```python
from build123d import *

# Parameters (mm, degrees)
SKETCH1_R           = 27
BOSS_EXTRUDE1_DEPTH = 5
SKETCH2_R           = 10
BOSS_EXTRUDE2_DEPTH = 2.5
CUT_EXTRUDE1_DEPTH  = 9


with BuildPart() as part:
    # Sketch1 → Boss-Extrude1 (new, symmetric)
    with BuildSketch(Plane.XY):
        Circle(SKETCH1_R)
    extrude(amount=BOSS_EXTRUDE1_DEPTH, both=True)

    # Sketch2 → Boss-Extrude2 (add)
    with BuildSketch(Plane(origin=(0, 0, -5), x_dir=(-1, 0, 0), z_dir=(0, 0, -1))):
        Circle(SKETCH2_R)
    extrude(amount=BOSS_EXTRUDE2_DEPTH)

    # Sketch3 → Cut-Extrude1 (cut)
    with BuildSketch(Plane(origin=(0, 0, -7.5), x_dir=(-1, 0, 0), z_dir=(0, 0, -1))):
        with BuildLine():
            Line((-1.953362486, -1.9), (1.953362486, -1.9))
            ThreePointArc((1.953362486, -1.9), (2.725, 0), (1.953362486, 1.9))
            Line((1.953362486, 1.9), (-1.953362486, 1.9))
            ThreePointArc((-1.953362486, 1.9), (-2.725, 0), (-1.953362486, -1.9))
        make_face()
    extrude(amount=-CUT_EXTRUDE1_DEPTH, mode=Mode.SUBTRACT)


solid = part.part
```
Check sheet for the modelled part. Datum: model origin and axes. Units: mm. A direction names the side the tool comes from. Round coordinates to 2 decimals unless told otherwise and drop trailing zeros. Order: outer loops, then holes, each group sorted by start corner. A loop starts at its lowest first (then second) coordinate and runs counter-clockwise, first axis right, second up. Notation, with made-up numbers: M -26.75,-0.75 L -3.75,-0.75 A20 ccw -3.75,25.25 Z; hole C 85.25,38.25 d6. An arc over 180 degrees is marked long. Answer in a Markdown table with one row per item.
(1) Draft check along Y on faces 3 (the flat face through (12, 0, -5)), 4 (the cylindrical face through (2.725, 0.029, -3.063)), 5 (the cylindrical face through (-5.85, -26.36, 0.07)). Enter one of: +Y half, -Y half, draft (parallel to the pull), parting line (faces both ways), or undercut.
Findings:
| item | result |
|---|---|
| face 3 | draft |
| face 4 | undercut |
| face 5 | parting line |
(2) Material ranges on line 1 along Z through (x, y) = (1.5, 10.5); line 2 along Y through (x, z) = (2, -3.5); line 3 along Y through (x, z) = (-1.5, -6), recorded low to high. Write a range as from..to.
Findings:
| item | result |
|---|---|
| line 1 | z = -5..5 |
| line 2 | y = -26.93..-1.85, 1.85..26.93 |
| line 3 | y = -9.89..-1.9, 1.9..9.89 |
(3) Section check A-A on z = -4.25. Record the boundary of the cut face in (x, y) (3 decimals), plus the area to 3 significant figures.
Findings:
| item | result |
|---|---|
| outline | C 0,0 d54; hole M -1.953,-1.9 L 1.953,-1.9 A2.725 ccw 1.953,1.9 L -1.953,1.9 A2.725 ccw Z |
| area | 2,270 mm^2 |
(4) Set-up check for faces 1 (the flat face through (0.1, -2.1, -7.5)), 2 (the flat face through (0, -1.9, -3)): record each of +Z, -Z, +X, -X, +Y, -Y from which the full face is reachable in a straight line by a thin tool's end or side.
Findings:
| item | result |
|---|---|
| face 1 | -Z, +X, -X, +Y, -Y |
| face 2 | -Z |
(5) Gauge pin test, flat ends, axial feed: pin 1 (4.5 mm diameter, centred on x = 0, z = -3.5, fed in from -Y); pin 2 (5 mm diameter, centred on x = -10, z = 0.5, fed in from -Y); pin 3 (6 mm diameter, centred on x = -13, z = 0, fed in from +Y). Record the tip position at first contact, or that the pin passes through.
Findings:
| item | result |
|---|---|
| pin 1 | stops at y = -27 |
| pin 2 | stops at y = -25.94 |
| pin 3 | stops at y = 25.08 |
(6) Section check B-B on y = 0. Record the boundary of the cut face in (x, z) (3 decimals), plus the area to 3 significant figures.
Findings:
| item | result |
|---|---|
| outline | M -27,-5 L -10,-5 L -10,-7.5 L -2.725,-7.5 L -2.725,1.5 L 2.725,1.5 L 2.725,-7.5 L 10,-7.5 L 10,-5 L 27,-5 L 27,5 L -27,5 Z |
| area | 541 mm^2 |
(7) Section check C-C on x = 0. Record the boundary of the cut face in (y, z).
Findings:
| item | result |
|---|---|
| outline | M -27,-5 L -10,-5 L -10,-7.5 L -1.9,-7.5 L -1.9,1.5 L 1.9,1.5 L 1.9,-7.5 L 10,-7.5 L 10,-5 L 27,-5 L 27,5 L -27,5 Z |
(8) Section check D-D on z = 3.25. Record the boundary of the cut face in (x, y).
Findings:
| item | result |
|---|---|
| outline | C 0,0 d54 |
